Could you check a few things on this model? Use its own coordinates, in mm. A direction names the side the tool comes from. Round coordinates to 2 decimals unless told otherwise and drop trailing zeros. Loops run counter-clockwise (first coordinate to the right, second up) from the corner with the lowest first, then second, coordinate; pieces in that order, holes last. Notation, with made-up numbers: (-13.5, 34) -> (15.5, 34) arc R10 cw to (15.5, 41) -> close; hole circle Ø6 at (-40, 10.25). An arc over 180 degrees is marked (long way). One line per item, written item: value.
```python
from build123d import *

# Parameters (mm, degrees)
SKETCH1_W           = 508
SKETCH1_H           = 228.6
BOSS_EXTRUDE1_DEPTH = 127
CUT_EXTRUDE1_DEPTH  = 114.3
SKETCH3_R           = 88.9
CUT_EXTRUDE2_DEPTH  = 157.988
SKETCH4_R           = 25.4
CUT_EXTRUDE3_DEPTH  = 157.988


with BuildPart() as part:
    # Sketch1 → Boss-Extrude1 (new body)
    with BuildSketch(Plane.XY):
        with Locations((-254, -114.3)):
            Rectangle(SKETCH1_W, SKETCH1_H)
    extrude(amount=BOSS_EXTRUDE1_DEPTH)

    # Sketch2 → Cut-Extrude1 (cut)
    with BuildSketch(Plane.XY.offset(127)):
        Polygon((-14.111111111, -6.35), (-254, -114.3), (-14.111111111, -222.25), (-6.35, -222.25), (-6.35, -6.35), align=None)
        Polygon((-14.111111111, -6.35), (-493.888888889, -6.35), (-254, -114.3), align=None)
        Polygon((-254, -114.3), (-493.888888889, -6.35), (-501.65, -6.35), (-501.65, -222.25), (-493.888888889, -222.25), align=None)
        Polygon((-14.111111111, -222.25), (-254, -114.3), (-493.888888889, -222.25), align=None)
    extrude(amount=-CUT_EXTRUDE1_DEPTH, mode=Mode.SUBTRACT)

    # Sketch3 → Cut-Extrude2 (cut)
    with BuildSketch(Plane.XY.offset(127)):
        with Locations((-254, -114.3)):
            Circle(SKETCH3_R)
    extrude(amount=-CUT_EXTRUDE2_DEPTH, mode=Mode.SUBTRACT)

    # Sketch4 → Cut-Extrude3 (cut)
    with BuildSketch(Plane(origin=(0, 0, 0), x_dir=(1, 0, 0), z_dir=(0, 1, 0))):
        with BuildLine():
            Line((-320.23493056, -38.112662334), (-474.665471548, -38.314758497))
            ThreePointArc((-474.665471548, -38.314758497), (-499.850713051, -63.5), (-474.665471548, -88.685241503))
            Line((-474.665471548, -88.685241503), (-320.23493056, -88.887337666))
            Line((-320.23493056, -88.887337666), (-320.168483959, -88.887424622))
            ThreePointArc((-320.168483959, -88.887424622), (-294.781059337, -63.5), (-320.168483959, -38.112575378))
            Line((-320.168483959, -38.112575378), (-320.23493056, -38.112662334))
        make_face()
        with Locations(Location((-127, -63.5, 0), (0, 0, 270))):
            Circle(SKETCH4_R)
    extrude(amount=-CUT_EXTRUDE3_DEPTH, mode=Mode.SUBTRACT)


solid = part.part
```
Item 1: If we mould it in two halves opening along Y, with no side actions, what happens to faces 1 (the face through (-501.65, -113, 71)), 2 (the face through (-258, -228.6, 63)), 3 (the face through (-258, 0, 63))? For each: released by +Y, released by -Y, zero draft, split by the parting line, or undercut.
Output:
face 1: undercut
face 2: released by -Y
face 3: released by +Y
Item 2: Will this pin go through, and if not, where does the flat tip stop? pin 1 Ø8 at (x, z) = (-302, 56) entering from +Y.
Output:
pin 1: stops at y = -222.25
Item 3: If we section it at B-B on z = 107.5: List the corners of the cut face in (x, y) for me, plus the area to 3 significant figures.
Output:
outline: (-508, -228.6) -> (0, -228.6) -> (0, 0) -> (-508, 0) -> close; hole (-501.65, -222.25) -> (-6.35, -222.25) -> (-6.35, -6.35) -> (-501.65, -6.35) -> close
area: 9,190 mm²
Item 4: I need wall thicknesses on line 1 (X direction, y = -4.25, z = 63.5); line 2 (Y direction, x = -254, z = 5.25); line 3 (Y direction, x = -99, z = 98). Which ranges of each line are inside material? Lowest first, please. Write a range as from..to.
Output:
line 1: x = -508..-499.85, -294.78..-152.4, -101.6..0
line 2: y = -228.6..-203.2, -25.4..0
line 3: y = -228.6..-222.25, -6.35..0
Item 5: If we section it at A-A on x = -127: List the corners of the cut face in (y, z) for me.
Output:
outline: (-228.6, 0) -> (0, 0) -> (0, 38.1) -> (-6.35, 38.1) -> (-6.35, 12.7) -> (-222.25, 12.7) -> (-222.25, 127) -> (-228.6, 127) -> close; (-6.35, 88.9) -> (0, 88.9) -> (0, 127) -> (-6.35, 127) -> close
Item 6: If we section it at C-C on z = 63.5: List the corners of the cut face in (x, y) for me, plus the area to 3 significant figures.
Output:
outline: (-508, -228.6) -> (0, -228.6) -> (0, 0) -> (-101.6, 0) -> (-101.6, -6.35) -> (-6.35, -6.35) -> (-6.35, -222.25) -> (-501.65, -222.25) -> (-501.65, -6.35) -> (-499.85, -6.35) -> (-499.85, 0) -> (-508, 0) -> close; (-294.78, -6.35) -> (-152.4, -6.35) -> (-152.4, 0) -> (-294.78, 0) -> close
area: 7,570 mm²
Item 7: If we section it at D-D on y = -161.5: List the corners of the cut face in (x, z) for me.
Output:
outline: (-508, 0) -> (-329.34, 0) -> (-329.34, 12.7) -> (-501.65, 12.7) -> (-501.65, 127) -> (-508, 127) -> close; (-178.66, 0) -> (0, 0) -> (0, 127) -> (-6.35, 127) -> (-6.35, 12.7) -> (-178.66, 12.7) -> close
Item 8: For faces 4 (the face through (-119.371, -3.131, 87.727)), 5 (the face through (-195, -6.35, 71)), 6 (the face through (-508, -116, 63)), which set-ups out of +Z, -Z, +X, -X, +Y, -Y let a thin tool reach every point of the face, with its end or its side?
Output:
face 4: +Y
face 5: +Z
face 6: +Z, -Z, -X, +Y, -Y
